```python
from build123d import *

# Parameters (mm, degrees)
SKETCH_1_W          = 95
SKETCH_1_H          = 70
EXTRUDE_1_DEPTH     = 3
SKETCH_2_R          = 3.5
EXTRUDE_2_DEPTH     = 8
SKETCH_3_R          = 1.5
CUT_EXTRUDE_1_DEPTH = 8
CHAMFER_2_SIZE      = 3
CHAMFER_2_SIZE_2    = 8
SKETCH_6_W          = 95
SKETCH_6_H          = 70
SKETCH_6_W_2        = 89
SKETCH_6_H_2        = 64
EXTRUDE_3_DEPTH     = 35
SKETCH_8_W          = 6
SKETCH_8_H          = 6
EXTRUDE_4_DEPTH     = 35
FILLET_4_R          = 1.5
SKETCH_10_R         = 1.5
CUT_EXTRUDE_2_DEPTH = 15
FILLET_6_R          = 3
SKETCH_11_R         = 6
CUT_EXTRUDE_3_DEPTH = 15
SKETCH_12_W         = 10
SKETCH_12_H         = 10
CUT_EXTRUDE_4_DEPTH = 15
FILLET_9_R          = 2.5
FILLET_10_R         = 3


# Some blends are built 0.0001 mm under size
with BuildPart() as part:
    # ｽｹｯﾁ1 → ﾎﾞｽ - 押し出し1 (new body)
    with BuildSketch(Plane.XY):
        with Locations((47.5, 35)):
            Rectangle(SKETCH_1_W, SKETCH_1_H)
    extrude(amount=EXTRUDE_1_DEPTH)

    # ｽｹｯﾁ2 → ﾎﾞｽ - 押し出し2 (add)
    with BuildSketch(Plane.XY.offset(3)):
        with Locations(Location((15, 55, 0), (0, 0, 180))):
            Circle(SKETCH_2_R)
        with Locations(Location((15, 15, 0), (0, 0, 180))):
            Circle(SKETCH_2_R)
        with Locations(Location((80, 55, 0), (0, 0, 180))):
            Circle(SKETCH_2_R)
        with Locations(Location((80, 15, 0), (0, 0, 180))):
            Circle(SKETCH_2_R)
    extrude(amount=EXTRUDE_2_DEPTH)

    # ｽｹｯﾁ3 → ｶｯﾄ - 押し出し1 (cut)
    with BuildSketch(Plane.XY.offset(11)):
        with Locations((15, 55)):
            Circle(SKETCH_3_R)
        with Locations((80, 55)):
            Circle(SKETCH_3_R)
        with Locations((15, 15)):
            Circle(SKETCH_3_R)
        with Locations((80, 15)):
            Circle(SKETCH_3_R)
    extrude(amount=-CUT_EXTRUDE_1_DEPTH, mode=Mode.SUBTRACT)

    # 面取り2
    # the kernel refuses this chamfer: 8, 3 mm, written as the material it adds along each edge
    with BuildSketch(Plane(origin=(15, 55, 3), x_dir=(-1, 0, 0), z_dir=(0, 1, 0))) as chamfer_2_piece_1_section:
        Polygon((3.5 + CHAMFER_2_SIZE, 0), (3.5, CHAMFER_2_SIZE_2), (3.5, 0), align=None)
    chamfer_2_piece_1 = revolve(axis=Axis((15, 55, 3), (0, 0, 1)), mode=Mode.PRIVATE)
    chamfer_2_piece_1 = split(chamfer_2_piece_1, bisect_by=Plane(origin=(19.987700919, 55, 11), z_dir=(0, 0, -1)), keep=Keep.TOP, mode=Mode.PRIVATE)
    add(chamfer_2_piece_1)
    with BuildSketch(Plane(origin=(15, 15, 3), x_dir=(-1, 0, 0), z_dir=(0, 1, 0))) as chamfer_2_piece_2_section:
        Polygon((3.5 + CHAMFER_2_SIZE, 0), (3.5, CHAMFER_2_SIZE_2), (3.5, 0), align=None)
    chamfer_2_piece_2 = revolve(axis=Axis((15, 15, 3), (0, 0, 1)), mode=Mode.PRIVATE)
    chamfer_2_piece_2 = split(chamfer_2_piece_2, bisect_by=Plane(origin=(19.987700919, 15, 11), z_dir=(0, 0, -1)), keep=Keep.TOP, mode=Mode.PRIVATE)
    add(chamfer_2_piece_2)
    with BuildSketch(Plane(origin=(80, 55, 3), x_dir=(-1, 0, 0), z_dir=(0, 1, 0))) as chamfer_2_piece_3_section:
        Polygon((3.5 + CHAMFER_2_SIZE, 0), (3.5, CHAMFER_2_SIZE_2), (3.5, 0), align=None)
    chamfer_2_piece_3 = revolve(axis=Axis((80, 55, 3), (0, 0, 1)), mode=Mode.PRIVATE)
    chamfer_2_piece_3 = split(chamfer_2_piece_3, bisect_by=Plane(origin=(84.987700919, 55, 11), z_dir=(0, 0, -1)), keep=Keep.TOP, mode=Mode.PRIVATE)
    add(chamfer_2_piece_3)
    with BuildSketch(Plane(origin=(80, 15, 3), x_dir=(-1, 0, 0), z_dir=(0, 1, 0))) as chamfer_2_piece_4_section:
        Polygon((3.5 + CHAMFER_2_SIZE, 0), (3.5, CHAMFER_2_SIZE_2), (3.5, 0), align=None)
    chamfer_2_piece_4 = revolve(axis=Axis((80, 15, 3), (0, 0, 1)), mode=Mode.PRIVATE)
    chamfer_2_piece_4 = split(chamfer_2_piece_4, bisect_by=Plane(origin=(84.987700919, 15, 11), z_dir=(0, 0, -1)), keep=Keep.TOP, mode=Mode.PRIVATE)
    add(chamfer_2_piece_4)

    # ｽｹｯﾁ6 → ﾎﾞｽ - 押し出し3 (add)
    with BuildSketch(Plane.XY.offset(3)):
        with Locations((47.5, 35)):
            Rectangle(SKETCH_6_W, SKETCH_6_H)
        with Locations((47.5, 35)):
            Rectangle(SKETCH_6_W_2, SKETCH_6_H_2, mode=Mode.SUBTRACT)
    extrude(amount=EXTRUDE_3_DEPTH)

    # ｽｹｯﾁ8 → ﾎﾞｽ - 押し出し4 (add)
    with BuildSketch(Plane.XY.offset(38)):
        with Locations((3, 67)):
            Rectangle(SKETCH_8_W, SKETCH_8_H)
        with Locations((92, 67)):
            Rectangle(SKETCH_8_W, SKETCH_8_H)
        with Locations((3, 3)):
            Rectangle(SKETCH_8_W, SKETCH_8_H)
        with Locations((92, 3)):
            Rectangle(SKETCH_8_W, SKETCH_8_H)
    extrude(amount=-EXTRUDE_4_DEPTH)

    # ﾌｨﾚｯﾄ4
    fillet_4_edges = [part.edges().sort_by_distance(p)[0] for p in [
        (92, 6, 20.5),
        (89, 6, 20.5),
        (89, 3, 20.5),
        (6, 3, 20.5),
        (6, 6, 20.5),
        (3, 6, 20.5),
        (92, 64, 20.5),
        (89, 64, 20.5),
        (89, 67, 20.5),
        (6, 64, 20.5),
        (6, 67, 20.5),
        (3, 64, 20.5),
    ]]
    fillet(fillet_4_edges, radius=FILLET_4_R - 0.0001)  # a hair under: the kernel refuses the full size

    # ｽｹｯﾁ10 → ｶｯﾄ - 押し出し2 (cut)
    with BuildSketch(Plane.XY.offset(38)):
        with Locations((3, 67)):
            Circle(SKETCH_10_R)
        with Locations((92, 67)):
            Circle(SKETCH_10_R)
        with Locations((3, 3)):
            Circle(SKETCH_10_R)
        with Locations((92, 3)):
            Circle(SKETCH_10_R)
    extrude(amount=-CUT_EXTRUDE_2_DEPTH, mode=Mode.SUBTRACT)

    # ﾌｨﾚｯﾄ6
    fillet_6_edges = [part.edges().sort_by_distance(p)[0] for p in [
        (0, 70, 19),
        (95, 70, 19),
        (95, 0, 19),
        (0, 0, 19),
    ]]
    fillet(fillet_6_edges, radius=FILLET_6_R)

    # ｽｹｯﾁ11 → ｶｯﾄ - 押し出し3 (cut)
    with BuildSketch(Plane(origin=(95, 0, 0), x_dir=(0, 0, -1), z_dir=(1, 0, 0))):
        with Locations((-21.599978, 44)):
            Circle(SKETCH_11_R)
    extrude(amount=-CUT_EXTRUDE_3_DEPTH, mode=Mode.SUBTRACT)

    # ｽｹｯﾁ12 → ｶｯﾄ - 押し出し4 (cut)
    with BuildSketch(Plane.XZ):
        with Locations((60.5, 33)):
            Rectangle(SKETCH_12_W, SKETCH_12_H)
    extrude(amount=-CUT_EXTRUDE_4_DEPTH, mode=Mode.SUBTRACT)

    # ﾌｨﾚｯﾄ9
    fillet_9_edges = [part.edges().sort_by_distance(p)[0] for p in [
        (65.5, 1.5, 28),
        (55.5, 1.5, 28),
    ]]
    fillet(fillet_9_edges, radius=FILLET_9_R)

    # ﾌｨﾚｯﾄ10
    fillet_10_edges = [part.edges().sort_by_distance(p)[0] for p in [
        (47.5, 0, 0),
        (0, 35, 0),
        (47.5, 70, 0),
        (95, 35, 0),
        (0.878679656, 69.121320344, 0),
        (94.121320344, 69.121320344, 0),
        (94.121320344, 0.878679656, 0),
        (0.878679656, 0.878679656, 0),
    ]]
    fillet(fillet_10_edges, radius=FILLET_10_R)


solid = part.part
```
Could you check a few things on this model? Use its own coordinates, in mm. A direction names the side the tool comes from. Give positions to 0.01 mm unless a question says otherwise; leave off trailing zeros. Order: outer loops, then holes, each group sorted by start corner. A loop starts at its lowest first (then second) coordinate and runs counter-clockwise, first axis right, second up.
Q1. I'm going to push flat-ended pins straight in: P1, Ø2.5, axis at x = 15, y = 55, coming from the +Z side; P2, Ø2.5, axis at x = 3.5, y = 3, coming from the +Z side; P3, Ø5.5, axis at x = 80.5, y = 53.5, coming from the +Z side; P4, Ø2.5, axis at y = 1, z = 35.5, coming from the +X side. Where does each tip first touch, or does it pass through?
Q2. Suppose I cut it at D-D, the plane z = 35.5. Count the separate pieces of the cut face and the enclosed holes in it, and give its area (3 significant figures).
Q3. Suppose I cut it at B-B, the plane x = 68.5. Write out the boundary of the cut face in (y, z).
Q4. For faces 1 (the cylindrical face through (81.43, 55.45, 7.06)), 2 (the flat face through (65.5, 1, 34)), 3 (the flat face through (95, 35, 20)), which set-ups out of +Z, -Z, +X, -X, +Y, -Y let a thin tool reach every point of the face, with its end or its side?
Q5. If I drill on line 1 along X through (y, z) = (53, 22); line 2 along Y through (x, z) = (36, 22); line 3 along Y through (x, z) = (15, 8) (3 decimals), over which ranges is the centre line in solid material (lowest first)?
Q6. Suppose I cut it at A-A, the plane y = 44. Write out the boundary of the cut face in (x, z), and give its area (3 significant figures).
Q7. Suppose I cut it at C-C, the plane y = 15. Write out the boundary of the cut face in (x, z), and give its area (3 significant figures).
Q8. We'd pull the mould along X, two halves only. Please class faces 4 (the flat face through (44, 69, 38)), 5 (the cylindrical face through (94.1, 0.86, 20.74)), 6 (the cylindrical face through (3.69, 1.67, 30.6)), 7 (the flat face through (55.5, 1, 34)): +X half, -X half, draft (parallel to the pull), parting line (faces both ways), or undercut.
Solution:
1. P1: stops at z = 3
1. P2: stops at z = 38
1. P3: stops at z = 11
1. P4: stops at x = 94.9
2. separate pieces: 1
2. enclosed holes: 4
2. area: 926 mm2
3. outline: (0, 3) arc R3 ccw to (3, 0) - (67, 0) arc R3 ccw to (70, 3) - (70, 38) - (67, 38) - (67, 3) - (3, 3) - (3, 38) - (0, 38) - close
4. face 1: +Z
4. face 2: +Z, -Y
4. face 3: +Z, -Z, +X, +Y, -Y
5. line 1: x = 0 to 3, 92 to 95
5. line 2: y = 0 to 3, 67 to 70
5. line 3: y = 0 to 3, 10.375 to 13.5, 16.5 to 19.625, 50.375 to 53.5, 56.5 to 59.625, 67 to 70
6. outline: (0, 3) arc R3 ccw to (3, 0) - (92, 0) arc R3 ccw to (95, 3) - (95, 15.6) - (92, 15.6) - (92, 3) - (3, 3) - (3, 38) - (0, 38) - close; (92, 27.6) - (95, 27.6) - (95, 38) - (92, 38) - close
6. area: 455 mm2
7. outline: (0, 3) arc R3 ccw to (3, 0) - (92, 0) arc R3 ccw to (95, 3) - (95, 38) - (92, 38) - (92, 3) - (86.5, 3) - (83.5, 11) - (81.5, 11) - (81.5, 3) - (78.5, 3) - (78.5, 11) - (76.5, 11) - (73.5, 3) - (21.5, 3) - (18.5, 11) - (16.5, 11) - (16.5, 3) - (13.5, 3) - (13.5, 11) - (11.5, 11) - (8.5, 3) - (3, 3) - (3, 38) - (0, 38) - close
7. area: 603 mm2
8. face 4: draft
8. face 5: +X half
8. face 6: undercut
8. face 7: undercut
